Print and shaded views of the part. All mm, measured from the part's lowest x, y and z. Round coordinates to 2 decimals unless told otherwise and drop trailing zeros. Loops run counter-clockwise (first coordinate to the right, second up) from the corner with the lowest first, then second, coordinate; pieces in that order, holes last. Notation, with made-up numbers: (-2, 8) - (34, 8) arc R23 cw to (34, 39) - close; hole circle Ø7 at (61.25, 26.5). An arc over 180 degrees is marked (long way). Answer as a JSON object with one key per item and string values.
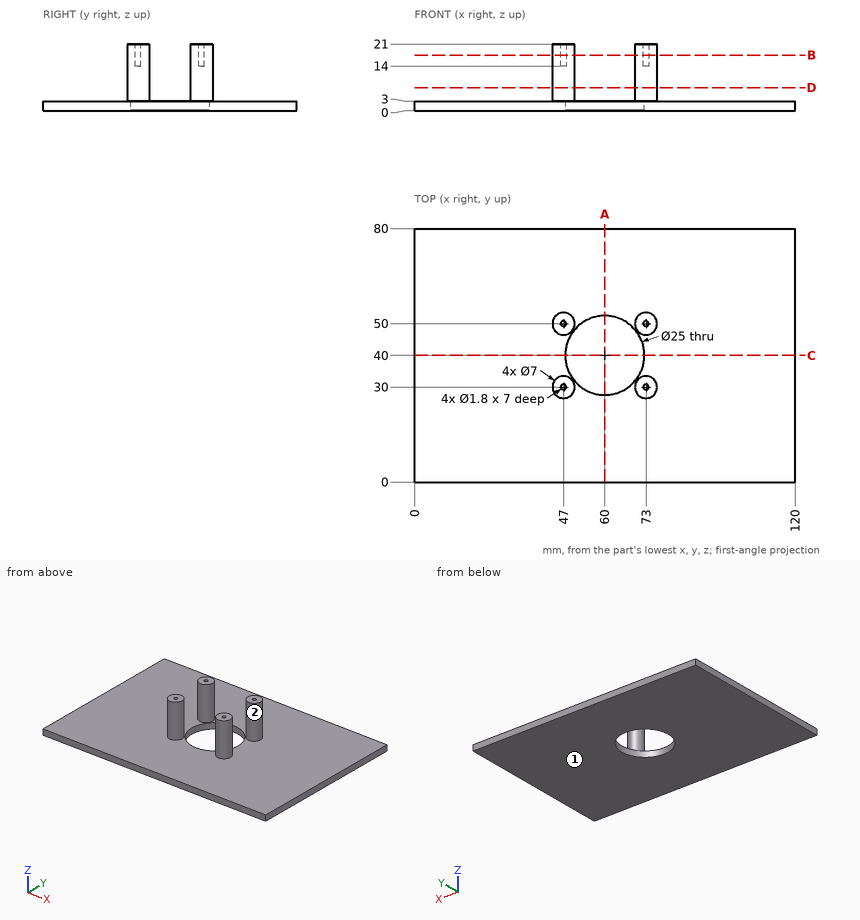
1) Slice it at B-B on z = 17.5. List the corners of the cut face in (x, y).
Values follow:
{"outline": "circle Ø7 at (47, 30); circle Ø7 at (47, 50); circle Ø7 at (73, 30); circle Ø7 at (73, 50); hole circle Ø1.8 at (47, 30); hole circle Ø1.8 at (47, 50); hole circle Ø1.8 at (73, 30); hole circle Ø1.8 at (73, 50)"}
2) Slice it at D-D on z = 7.25. List the corners of the cut face in (x, y), then the cut area to 3 significant figures.
Values follow:
{"outline": "circle Ø7 at (47, 30); circle Ø7 at (47, 50); circle Ø7 at (73, 30); circle Ø7 at (73, 50)", "area": "154 mm²"}
3) Slice it at C-C on y = 40. List the corners of the cut face in (x, z).
Values follow:
{"outline": "(0, 0) - (47.5, 0) - (47.5, 3) - (0, 3) - close; (72.5, 0) - (120, 0) - (120, 3) - (72.5, 3) - close"}
4) Two-plate mould, pull along X, no slides. Class the marked faces 1 and 2: pulls with the +X half, pulls with the -X half, needs draft (parallel to the pull), parting line crosses it, or undercut.
Values follow:
{"face 1": "needs draft", "face 2": "undercut"}
5) Drop flat-ended pins along their axis: P1, Ø3, axis at x = 23.5, z = 5.5, coming from the -Y side; P2, Ø6, axis at y = 55.5, z = 18, coming from the +X side; P3, Ø1, axis at x = 80.5, y = 42.5, coming from the +Z side; P4, Ø0.5, axis at x = 73, y = 50.5, coming from the +Z side. Give the stop position or say it passes through.
Values follow:
{"P1": "through", "P2": "x = 75.45", "P3": "z = 3", "P4": "z = 14"}
6) Probe probe 1 along Y at (x, z) = (47, 17.5); probe 2 along Y at (x, z) = (60, 2.2); probe 3 along Z at (x, y) = (8.5, 25.5). List the from-to ranges inside material, lowest first.
Values follow:
{"probe 1": "26.5 to 29.1, 30.9 to 33.5, 46.5 to 49.1, 50.9 to 53.5", "probe 2": "0 to 27.5, 52.5 to 80", "probe 3": "0 to 3"}
7) Slice it at A-A on x = 60. List the corners of the cut face in (y, z), then the cut area to 3 significant figures.
Values follow:
{"outline": "(0, 0) - (27.5, 0) - (27.5, 3) - (0, 3) - close; (52.5, 0) - (80, 0) - (80, 3) - (52.5, 3) - close", "area": "165 mm²"}
